Source: three-view drawing plus pictorial views. Frame: mm from the lowest corner of the part. A direction names the side the tool comes from. Round coordinates to 2 decimals unless told otherwise and drop trailing zeros. Write each loop counter-clockwise with the first axis right and the second up, starting at its lowest first coordinate (ties: lowest second). Pieces come first, ordered by that corner, then holes. Notation, with made-up numbers: M 20.25,9.25 L 39.25,9.25 A23 ccw 39.25,37.25 Z; hole C 74,16 d9. An arc over 180 degrees is marked long. Answer as CSV lines item,"result". Start each with the question number.
Q1. First-contact query: pin 1 (3 mm diameter, centred on x = 24.5, z = 4, fed in from +Y); pin 2 (6 mm diameter, centred on y = 25.5, z = 2, fed in from -X); pin 3 (1.5 mm diameter, centred on y = 9, z = 1.5, fed in from +X); pin 4 (4 mm diameter, centred on x = 15.5, z = 7.5, fed in from -Y). Flat tips, straight axial feed; report the tip coordinate or a pass-through.
Q2. Section query C-C on x = 18.5. Output: boundary loops of the cut face in (y, z), and give its area (3 significant figures).
Q3. Reachability of the marked faces 1, 2, 3 and 4 from +Z, -Z, +X, -X, +Y, -Y: full face, straight path, thin tool, end or side. Return the list, or none.
Q4. Section query B-B on z = 7. Give the number of separate pieces and of enclosed holes in the cut face, and give its area (3 significant figures).
Q5. Section query A-A on x = 1.65. Output: boundary loops of the cut face in (y, z), and give its area (3 significant figures).
Q6. Section query D-D on y = 3. Output: boundary loops of the cut face in (x, z), and give its area (3 significant figures).
Q7. Ray query, probe 1 along Z at (x, y) = (28.25, 15.8); probe 2 along Y at (x, z) = (5, 5.5); probe 3 along Y at (x, z) = (23.75, 5.5). Return the intervals inside material, ascending.
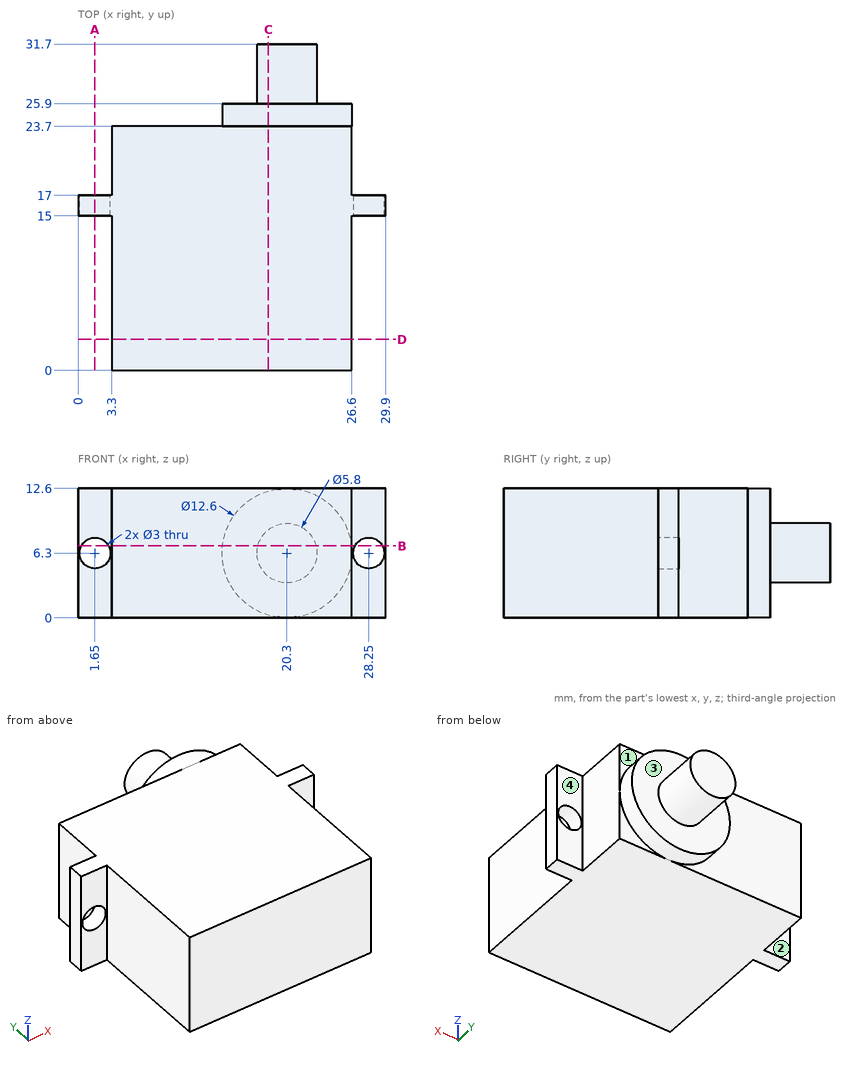
Entries:
1,pin 1,"stops at y = 25.9"
1,pin 2,"stops at x = 3.3"
1,pin 3,"stops at x = 26.6"
1,pin 4,"stops at y = 0"
2,outline,"M 0,0 L 23.7,0 L 23.7,0.26 L 25.9,0.26 L 25.9,4.03 L 31.7,4.03 L 31.7,8.57 L 25.9,8.57 L 25.9,12.34 L 23.7,12.34 L 23.7,12.6 L 0,12.6 Z"
2,area,"352 mm^2"
3,face 1,"+Z, +X, +Y"
3,face 2,"+Z, -Z, -X, +Y"
3,face 3,"+Y"
3,face 4,"+Z, -Z, +X, +Y"
4,separate pieces,"3"
4,enclosed holes,"0"
4,area,"615 mm^2"
5,outline,"M 15,0 L 17,0 L 17,4.8 L 15,4.8 Z; M 15,7.8 L 17,7.8 L 17,12.6 L 15,12.6 Z"
5,area,"19.2 mm^2"
6,outline,"M 3.3,0 L 26.6,0 L 26.6,12.6 L 3.3,12.6 Z"
6,area,"294 mm^2"
7,probe 1,"z = 0 to 4.8, 7.8 to 12.6"
7,probe 2,"y = 0 to 23.7"
7,probe 3,"y = 0 to 25.9"
